```python
from build123d import *

# Parameters (mm, degrees)
SKETCH_1_W           = 57
SKETCH_1_H           = 16
EXTRUDE_1_DEPTH      = 5
FILLET_1_R           = 1.5
HOLE_WIZARD_M41_D    = 4.5
CHAMFER_1_SIZE       = 1.5
SKETCH_2_R           = 4.25
CUT_EXTRUDE_1_DEPTH  = 1
SKETCH_7_R           = 3.5
CUT_EXTRUDE_2_DEPTH  = 60.338014797
EXTRUDE_2_DEPTH      = 13
EXTRUDE_2_DEPTH_BACK = 13
SKETCH_10_R          = 3.5
EXTRUDE_3_DEPTH      = 6
SKETCH_11_R          = 2.25
CUT_EXTRUDE_3_DEPTH  = 9.25
EXTRUDE_START        = 0.1
SKETCH_12_R          = 4
SKETCH_12_R_2        = 2.25
EXTRUDE_4_DEPTH      = 0.1
SKETCH_13_R          = 1.75
CUT_EXTRUDE_4_DEPTH  = 5


with BuildPart() as part:
    # Sketch 1 → Extrude 1 (new body)
    with BuildSketch(Plane(origin=(0, 0, 0), x_dir=(1, 0, 0), z_dir=(0, 1, 0))):
        with Locations((28.5, 8)):
            Rectangle(SKETCH_1_W, SKETCH_1_H)
    extrude(amount=EXTRUDE_1_DEPTH)

    # Fillet 1
    fillet_1_edges = [part.edges().sort_by_distance(p)[0] for p in [
        (0, 5, -8),
        (28.5, 5, 0),
        (57, 5, -8),
        (0, 2.5, 0),
        (0, 2.5, -16),
        (57, 2.5, -16),
        (57, 2.5, 0),
    ]]
    fillet(fillet_1_edges, radius=FILLET_1_R)

    # Hole Wizard M41 (through all)
    with Locations(Plane(origin=(0, 5, 0), x_dir=(1, 0, 0), z_dir=(0, 1, 0))):
        with Locations((6.25, 8), (50.75, 8)):
            Hole(HOLE_WIZARD_M41_D / 2)

    # Chamfer 1
    chamfer_1_edges = [part.edges().sort_by_distance(p)[0] for p in [
        (53, 5, -8),
        (8.5, 5, -8),
    ]]
    chamfer(chamfer_1_edges, length=CHAMFER_1_SIZE)

    # Sketch 2 → Cut-Extrude 1 (cut)
    with BuildSketch(Plane(origin=(0, 5, 0), x_dir=(1, 0, 0), z_dir=(0, 1, 0))):
        with Locations(Location((18.625, 8, 0), (0, 0, 270))):
            Circle(SKETCH_2_R)
        with Locations(Location((38.375, 8, 0), (0, 0, 270))):
            Circle(SKETCH_2_R)
    extrude(amount=-CUT_EXTRUDE_1_DEPTH, mode=Mode.SUBTRACT)

    # Sketch 7 → Cut-Extrude 2 (cut, through all)
    with BuildSketch(Plane(origin=(0, 4, 0), x_dir=(1, 0, 0), z_dir=(0, 1, 0))):
        with Locations(Location((18.625, 8, 0), (0, 0, 270))):
            Circle(SKETCH_7_R)
        with Locations(Location((38.375, 8, 0), (0, 0, 270))):
            Circle(SKETCH_7_R)
    extrude(amount=-CUT_EXTRUDE_2_DEPTH, mode=Mode.SUBTRACT)

    # Sketch 9 → Extrude 2 (add, two sides: drawn at the far end of the back side and taken through both)
    with BuildSketch(Plane.ZY.offset(-28.5).offset(-EXTRUDE_2_DEPTH_BACK)):
        Polygon((-19, 5), (-28, 0), (-25.3, 0), (-19, 3.5), (-16, 3.5), (-16, 5), align=None)
    extrude(amount=EXTRUDE_2_DEPTH + EXTRUDE_2_DEPTH_BACK)

    # Sketch 10 → Extrude 3 (add)
    with BuildSketch(Plane.XZ):
        with BuildLine():
            Line((18.5, -13.5), (38.5, -13.5))
            ThreePointArc((38.5, -13.5), (44, -8), (38.5, -2.5))
            Line((38.5, -2.5), (18.5, -2.5))
            ThreePointArc((18.5, -2.5), (13, -8), (18.5, -13.5))
        make_face()
        with Locations(Location((38.375, -8, 0), (0, 0, 90))):
            Circle(SKETCH_10_R, mode=Mode.SUBTRACT)
        with Locations(Location((18.625, -8, 0), (0, 0, 90))):
            Circle(SKETCH_10_R, mode=Mode.SUBTRACT)
    extrude(amount=EXTRUDE_3_DEPTH)

    # Sketch 11 → Cut-Extrude 3 (cut)
    with BuildSketch(Plane.XZ.offset(6)):
        with Locations(Location((28.5, -8, 0), (0, 0, 270))):
            Circle(SKETCH_11_R)
    extrude(amount=-CUT_EXTRUDE_3_DEPTH, mode=Mode.SUBTRACT)

    # Sketch 12 → Extrude 4 (add)
    with BuildSketch(Plane.XZ.offset(6).offset(EXTRUDE_START)):
        with Locations(Location((28.5, -8, 0), (0, 0, 270))):
            Circle(SKETCH_12_R)
        with Locations(Location((28.5, -8, 0), (0, 0, 270))):
            Circle(SKETCH_12_R_2, mode=Mode.SUBTRACT)
    extrude(amount=-EXTRUDE_4_DEPTH)

    # Sketch 13 → Cut-Extrude 4 (cut)
    with BuildSketch(Plane(origin=(0, 0, -13.5), x_dir=(-1, 0, 0), z_dir=(0, 0, -1))):
        with Locations((-38.375, -3)):
            Circle(SKETCH_13_R)
        with Locations((-18.625, -3)):
            Circle(SKETCH_13_R)
    extrude(amount=-CUT_EXTRUDE_4_DEPTH, mode=Mode.SUBTRACT)


solid = part.part
```
Work out the finished part from the listing and answer in its coordinate system (mm). A direction names the side the tool comes from. Coordinates: 2 decimals unless noted, no trailing zeros. Write each loop counter-clockwise with the first axis right and the second up, starting at its lowest first coordinate (ties: lowest second). Pieces come first, ordered by that corner, then holes.
Q1. Each of these flat-tipped pins is pushed along its axis until it touches: pin 1 Ø3.5 at (x, z) = (34.5, -17.5) entering from -Y; pin 2 Ø2 at (y, z) = (1, -25) entering from +X; pin 3 Ø5 at (x, z) = (6.25, -8) entering from +Y. Where does it stop, or does it pass through?
Q2. A cutting plane is placed at C-C, the plane x = 28.5. Give the vertices of the cut face in (y, z).
Q3. A cutting plane is placed at A-A, the plane x = 6.25. Give the vertices of the cut face in (y, z).
Q4. Find the intervals of material crossed by line 1 (X direction, y = 2.3, z = -8) (3 decimals); line 2 (X direction, y = 4.55, z = -8) (3 decimals); line 3 (X direction, y = 4.85, z = -8) (3 decimals), in increasing order.
Q5. A cutting plane is placed at B-B, the plane y = 1.75. Give the vertices of the cut face in (x, z) (3 decimals).
Q6. Determine the mould class of faces 1 (the face through (28.682, 2.535, -23.437)), 2 (the face through (53, 2, -8)), 3 (the face through (0.43, 1.77, -0.45)) for opening direction X: released by +X, released by -X, zero draft, split by the parting line, or undercut.
Q7. Which of the six approach directions +Z, -Z, +X, -X, +Y, -Y give full straight-line access (tool end or side, diameter ignored) to faces 4 (the face through (44, -3, -8)), 5 (the face through (26.304, -1.49, -7.512)), 6 (the face through (42.59, 4.51, -8.55))?
Q8. A cutting plane is placed at D-D, the plane z = -8. State how many separate pieces and enclosed holes the cut face has, then the cut area to 3 significant figures.
Findings below:
1. pin 1: stops at y = 0
1. pin 2: stops at x = 41.5
1. pin 3: stops at y = 3.75
2. outline: (-6.1, -12) - (-6, -12) - (-6, -13.5) - (0, -13.5) - (0, -16) - (3.5, -16) - (3.5, -19) - (0, -25.3) - (0, -28) - (5, -19) - (5, -1.5) arc R1.5 ccw to (3.5, 0) - (0, 0) - (0, -2.5) - (-6, -2.5) - (-6, -4) - (-6.1, -4) - (-6.1, -5.75) - (3.25, -5.75) - (3.25, -10.25) - (-6.1, -10.25) - close
3. outline: (0, -16) - (5, -16) - (5, -11.75) - (3.5, -10.25) - (0, -10.25) - close; (0, -5.75) - (3.5, -5.75) - (5, -4.25) - (5, -1.5) arc R1.5 ccw to (3.5, 0) - (0, 0) - close
4. line 1: x = 0 to 4, 8.5 to 15.125, 22.125 to 26.25, 30.75 to 34.875, 41.875 to 48.5, 53 to 57
4. line 2: x = 0.429 to 2.95, 9.55 to 14.375, 22.875 to 34.125, 42.625 to 47.45, 54.05 to 56.571
4. line 3: x = 0.846 to 2.65, 9.85 to 14.375, 22.875 to 34.125, 42.625 to 47.15, 54.35 to 56.154
5. outline: (0, -14.5) arc R1.5 ccw to (1.5, -16) - (55.5, -16) arc R1.5 ccw to (57, -14.5) - (57, -1.5) arc R1.5 ccw to (55.5, 0) - (1.5, 0) arc R1.5 ccw to (0, -1.5) - close; (15.5, -24.85) - (41.5, -24.85) - (41.5, -22.15) - (15.5, -22.15) - close; hole circle Ø4.5 at (6.25, -8); hole circle Ø7 at (18.625, -8); hole circle Ø4.5 at (28.5, -8); hole circle Ø7 at (38.375, -8); hole circle Ø4.5 at (50.75, -8)
6. face 1: zero draft
6. face 2: undercut
6. face 3: released by -X
7. face 4: +X, -Y
7. face 5: -Y
7. face 6: +Y
8. separate pieces: 5
8. enclosed holes: 0
8. area: 222 mm2
